Here's how the part is built. I have some questions about the finished solid (model axes, mm). Face numbers are marked on the shaded views. A direction names the side the tool comes from. Coordinates: 2 decimals unless noted, no trailing zeros. Loops run counter-clockwise (first coordinate to the right, second up) from the corner with the lowest first, then second, coordinate; pieces in that order, holes last. Notation, with made-up numbers: (-26.5, 9.25) -> (-18.5, 9.25) arc R7 ccw to (-18.5, 14.25) -> close; hole circle Ø8 at (0, -16). An arc over 180 degrees is marked (long way). Answer as a JSON object with one key per item and string values. Group by question number.
Q1. I'm going to push flat-ended pins straight in: pin 1 (19 mm diameter, centred on y = -17, z = 26.5, fed in from +X); pin 2 (6 mm diameter, centred on x = -11, y = -49, fed in from -Z); pin 3 (1 mm diameter, centred on x = 1, z = 13, fed in from +Y); pin 4 (1.2 mm diameter, centred on y = 29.5, z = 19, fed in from -X). Where does each tip first touch, or does it pass through?
Q2. I want a section at D-D on z = 33.5. Write out the boundary of the cut face in (x, y), then the cut area to 3 significant figures.
Q3. I want a section at B-B on x = 0. Write out the boundary of the cut face in (y, z).
Q4. On a 3-axis mill with a long thin cutter (end or side, diameter ignored), from which of +Z, -Z, +X, -X, +Y, -Y can I reach the whole of each face in a straight line? I mean the marked faces 5, 6 and 7. Say none if no direction works.
Q5. I need wall thicknesses on line 1 (Y direction, x = 11, z = 2); line 2 (X direction, y = -19, z = 15); line 3 (Z direction, x = -10.5, y = -41). Which ranges of each line are inside material? Lowest first, please.
Q6. I want a section at A-A on z = 6.5. Write out the boundary of the cut face in (x, y), then the cut area to 3 significant figures.
Q7. I want a section at C-C on y = 56.5. Write out the boundary of the cut face in (x, z).
Q8. Thinking about a two-plate mould opening in X: for the marked faces 1, 2, 3 and 4, which applies, released by +X, released by -X, zero draft, split by the parting line, or undercut?
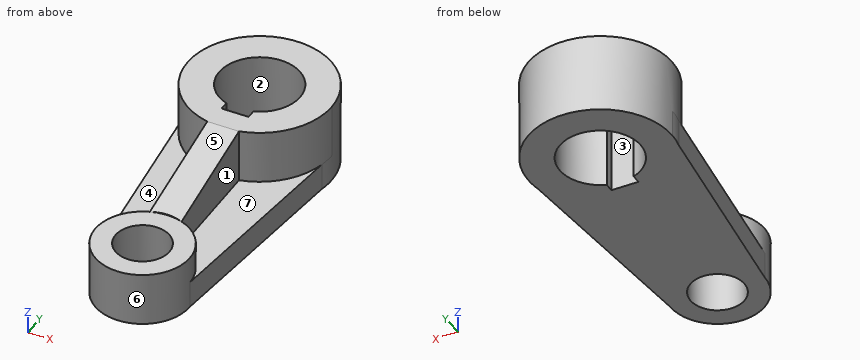
```python
from build123d import *

# Parameters (mm, degrees)
F0_R      = 9.477436644
F1_DEPTH  = 12
F2_R      = 32
F3_DEPTH  = 24
F4_R      = 21
F5_DEPTH  = 12
F7_DEPTH  = 36.001
F8_R      = 12
F9_DEPTH  = 24.001
F11_DEPTH = 24
F13_DEPTH = 25


with BuildPart() as f1:
    # F0 (on Top) → F1 (new body)
    with BuildSketch(Plane.XY):
        with BuildLine():
            ThreePointArc((-31.2348582156, 41.2315710582), (0, 16.187405462), (31.2348582156, 41.2315710582))
            Line((31.2348582156, 41.2315710582), (32, 48.187405462))
            ThreePointArc((32, 48.187405462), (0, 80.187405462), (-32, 48.187405462))
            Line((-32, 48.187405462), (-31.2348582156, 41.2315710582))
        make_face()
        with BuildLine():
            ThreePointArc((-6, 31.2168427135), (-10.3923048454, 62.8843439187), (18, 48.187405462))
            ThreePointArc((18, 48.187405462), (14.6969384567, 37.7951006165), (6, 31.2168427135))
            Line((6, 31.2168427135), (6, 28.187405462))
            Line((6, 28.187405462), (-6, 28.187405462))
            Line((-6, 28.187405462), (-6, 31.2168427135))
        make_face(mode=Mode.SUBTRACT)
        with BuildLine():
            ThreePointArc((-21, -51.812594538), (0, -30.812594538), (21, -51.812594538))
            Line((21, -51.812594538), (31.2348582156, 41.2315710582))
            ThreePointArc((31.2348582156, 41.2315710582), (0, 16.187405462), (-31.2348582156, 41.2315710582))
            Line((-31.2348582156, 41.2315710582), (-21, -51.812594538))
        make_face()
        with BuildLine():
            ThreePointArc((-21, -51.812594538), (0, -72.812594538), (21, -51.812594538))
            ThreePointArc((21, -51.812594538), (0, -30.812594538), (-21, -51.812594538))
        make_face()
        with Locations((0, -51.812594538)):
            Circle(F0_R, mode=Mode.SUBTRACT)
        with BuildLine():
            ThreePointArc((6, 31.2168427135), (14.6969384567, 37.7951006165), (18, 48.187405462))
            ThreePointArc((18, 48.187405462), (-10.3923048454, 62.8843439187), (-6, 31.2168427135))
            ThreePointArc((-6, 31.2168427135), (0, 30.187405462), (6, 31.2168427135))
        make_face()
        with Locations((0, -51.812594538)):
            Circle(F0_R)
        with BuildLine():
            ThreePointArc((6, 31.2168427135), (0, 30.187405462), (-6, 31.2168427135))
            Line((-6, 31.2168427135), (-6, 28.187405462))
            Line((-6, 28.187405462), (6, 28.187405462))
            Line((6, 28.187405462), (6, 31.2168427135))
        make_face()
        with BuildLine():
            ThreePointArc((-32, 48.187405462), (-31.8081393899, 44.6885101291), (-31.2348582156, 41.2315710582))
            Line((-31.2348582156, 41.2315710582), (-32, 48.187405462))
        make_face()
        with BuildLine():
            Line((32, 48.187405462), (31.2348582156, 41.2315710582))
            ThreePointArc((31.2348582156, 41.2315710582), (31.8081393899, 44.6885101291), (32, 48.187405462))
        make_face()
    extrude(amount=F1_DEPTH)

    # F2 (on face) → F3 (join)
    with BuildSketch(Plane.XY.offset(12)):
        with Locations((0, 48.187405462)):
            Circle(F2_R)
    extrude(amount=F3_DEPTH)

    # F4 (on face) → F5 (join)
    with BuildSketch(Plane.XY.offset(12)):
        with Locations((0, -51.812594538)):
            Circle(F4_R)
    extrude(amount=F5_DEPTH)

    # F6 (on face) → F7 (cut, through all)
    with BuildSketch(Plane.XY.offset(36)):
        with BuildLine():
            Line((6, 31.187405462), (5.9160797831, 31.187405462))
            ThreePointArc((5.9160797831, 31.187405462), (0, 66.187405462), (-5.9160797831, 31.187405462))
            Line((-5.9160797831, 31.187405462), (-6, 31.187405462))
            Line((-6, 31.187405462), (-6, 27.187405462))
            Line((-6, 27.187405462), (6, 27.187405462))
            Line((6, 27.187405462), (6, 31.187405462))
        make_face()
    extrude(amount=-F7_DEPTH, mode=Mode.SUBTRACT)

    # F8 (on face) → F9 (cut, through all)
    with BuildSketch(Plane.XY.offset(24)):
        with Locations((0, -51.812594538)):
            Circle(F8_R)
    extrude(amount=-F9_DEPTH, mode=Mode.SUBTRACT)

    # F10 (on face) → F11 (join)
    with BuildSketch(Plane.XY.offset(12)):
        with BuildLine():
            ThreePointArc((-7.0413727647, -32.0282808126), (0, -30.812594538), (7.0413727647, -32.0282808126))
            Line((7.0413727647, -32.0282808126), (7.0413727647, 16.9717191874))
            ThreePointArc((7.0413727647, 16.9717191874), (0, 16.187405462), (-7.0413727647, 16.9717191874))
            Line((-7.0413727647, 16.9717191874), (-7.0413727647, -32.0282808126))
        make_face()
    extrude(amount=F11_DEPTH)

    # F12 (on face) → F13 (cut)
    with BuildSketch(Plane.YZ.offset(7.0413727647)):
        Polygon((-32.0282808126, 36), (-32.0282808126, 24), (16.9717191874, 36), align=None)
    extrude(amount=-F13_DEPTH, mode=Mode.SUBTRACT)


solid = f1.part
```
Result set:
{
 "1": {"pin 1": "stops at x = 7.04", "pin 2": "stops at z = 0", "pin 3": "stops at y = 80.18", "pin 4": "stops at x = -26.4"},
 "2": {"outline": "(-7.04, 6.76) -> (7.04, 6.76) -> (7.04, 16.97) arc R32 ccw (long way) to (-7.04, 16.97) -> close; hole (-6, 27.19) -> (6, 27.19) -> (6, 31.19) -> (5.92, 31.19) arc R18 ccw (long way) to (-5.92, 31.19) -> (-6, 31.19) -> close", "area": "2,300 mm²"},
 "3": {"outline": "(-72.81, 0) -> (-63.81, 0) -> (-63.81, 24) -> (-72.81, 24) -> close; (-39.81, 0) -> (27.19, 0) -> (27.19, 36) -> (16.97, 36) -> (-30.81, 24.3) -> (-30.81, 24) -> (-39.81, 24) -> close; (66.19, 0) -> (80.19, 0) -> (80.19, 36) -> (66.19, 36) -> close"},
 "4": {"face 5": "+Z, +X, -X, -Y", "face 6": "+Z", "face 7": "+Z, +X"},
 "5": {"line 1": "y = -69.7 to -56.61, -47.02 to 33.94, 62.44 to 78.24", "line 2": "x = -7.04 to 7.04", "line 3": "z = 0 to 24"},
 "6": {"outline": "(-31.23, 41.23) -> (-21, -51.81) arc R21 ccw to (21, -51.81) -> (31.23, 41.23) arc R32 ccw (long way) to start; hole circle Ø24 at (0, -51.81); hole (-6, 27.19) -> (6, 27.19) -> (6, 31.19) -> (5.92, 31.19) arc R18 ccw (long way) to (-5.92, 31.19) -> (-6, 31.19) -> close", "area": "6,090 mm²"},
 "7": {"outline": "(-30.9, 0) -> (-15.97, 0) -> (-15.97, 36) -> (-30.9, 36) -> close; (15.97, 0) -> (30.9, 0) -> (30.9, 36) -> (15.97, 36) -> close"},
 "8": {"face 1": "released by +X", "face 2": "undercut", "face 3": "undercut", "face 4": "zero draft"}
}
